Can you work these out from the model? Positions are in its coordinate system, mm. Coordinates: 2 decimals unless noted, no trailing zeros. Loops run counter-clockwise (first coordinate to the right, second up) from the corner with the lowest first, then second, coordinate; pieces in that order, holes last.
```python
from build123d import *

# Parameters (mm, degrees)
F0_R     = 35
F0_R_2   = 3.771368
F1_DEPTH = 35
F2_DEPTH = 25


with BuildPart() as f1:
    # F0 (on Top) → F1 (new body)
    with BuildSketch(Plane.XY):
        Circle(F0_R)
        with Locations((-0.389893, -27.902429)):
            Circle(F0_R_2, mode=Mode.SUBTRACT)
        with Locations((-16.670046, -22.486003)):
            Circle(F0_R_2, mode=Mode.SUBTRACT)
        with Locations((-26.65727, -8.534788)):
            Circle(F0_R_2, mode=Mode.SUBTRACT)
        with Locations((15.964723, -22.715176)):
            Circle(F0_R_2, mode=Mode.SUBTRACT)
        with Locations((26.146894, -8.905599)):
            Circle(F0_R_2, mode=Mode.SUBTRACT)
        with Locations((-26.536787, 8.622325)):
            Circle(F0_R_2, mode=Mode.SUBTRACT)
        with Locations((-16.354616, 22.431902)):
            Circle(F0_R_2, mode=Mode.SUBTRACT)
        with Locations((26.267377, 8.251514)):
            Circle(F0_R_2, mode=Mode.SUBTRACT)
        with Locations((16.280153, 22.202729)):
            Circle(F0_R_2, mode=Mode.SUBTRACT)
        with Locations((0, 27.619155)):
            Circle(F0_R_2, mode=Mode.SUBTRACT)
    extrude(amount=F1_DEPTH)

    # F0 (on Top) → F2 (join)
    with BuildSketch(Plane.XY):
        Circle(F0_R)
        with Locations((-0.389893, -27.902429)):
            Circle(F0_R_2, mode=Mode.SUBTRACT)
        with Locations((-16.670046, -22.486003)):
            Circle(F0_R_2, mode=Mode.SUBTRACT)
        with Locations((-26.65727, -8.534788)):
            Circle(F0_R_2, mode=Mode.SUBTRACT)
        with Locations((15.964723, -22.715176)):
            Circle(F0_R_2, mode=Mode.SUBTRACT)
        with Locations((26.146894, -8.905599)):
            Circle(F0_R_2, mode=Mode.SUBTRACT)
        with Locations((-26.536787, 8.622325)):
            Circle(F0_R_2, mode=Mode.SUBTRACT)
        with Locations((-16.354616, 22.431902)):
            Circle(F0_R_2, mode=Mode.SUBTRACT)
        with Locations((26.267377, 8.251514)):
            Circle(F0_R_2, mode=Mode.SUBTRACT)
        with Locations((16.280153, 22.202729)):
            Circle(F0_R_2, mode=Mode.SUBTRACT)
        with Locations((0, 27.619155)):
            Circle(F0_R_2, mode=Mode.SUBTRACT)
    extrude(amount=F2_DEPTH)


solid = f1.part
```
(1) I'm going to push flat-ended pins straight in: pin 1 (4 mm diameter, centred on y = -3, z = 6.5, fed in from +X); pin 2 (1.5 mm diameter, centred on x = -2.5, z = 30, fed in from +Y); pin 3 (5 mm diameter, centred on x = 2.5, z = 14, fed in from -Y). Where does each tip first touch, or does it pass through?
Check values:
pin 1: stops at x = 34.99
pin 2: stops at y = 34.96
pin 3: stops at y = -35
(2) I want a section at A-A on x = -14.5. Write out the boundary of the cut face in (y, z), then the cut area to 3 significant figures.
Check values:
outline: (-31.86, 0) - (-25.57, 0) - (-25.57, 35) - (-31.86, 35) - close; (-19.4, 0) - (19.15, 0) - (19.15, 35) - (-19.4, 35) - close; (25.72, 0) - (31.86, 0) - (31.86, 35) - (25.72, 35) - close
area: 1,780 mm2
(3) If I drill on probe 1 along Y at (x, z) = (0, 21); probe 2 along X at (y, z) = (11.5, 3); probe 3 along Y at (x, z) = (-16, 13), over which ranges is the centre line in solid material (lowest first)?
Check values:
probe 1: y = -35 to -31.65, -24.15 to 23.85, 31.39 to 35
probe 2: x = -33.06 to -28.97, -24.1 to 24.35, 28.18 to 33.06
probe 3: y = -31.13 to -26.2, -18.77 to 18.68, 26.19 to 31.13
(4) I want a section at C-C on x = 0. Write out the boundary of the cut face in (y, z).
Check values:
outline: (-35, 0) - (-31.65, 0) - (-31.65, 35) - (-35, 35) - close; (-24.15, 0) - (23.85, 0) - (23.85, 35) - (-24.15, 35) - close; (31.39, 0) - (35, 0) - (35, 35) - (31.39, 35) - close
(5) I want a section at B-B on z = 7.5. State how many separate pieces and enclosed holes the cut face has, then the cut area to 3 significant figures.
Check values:
separate pieces: 1
enclosed holes: 10
area: 3,400 mm2
(6) I want a section at D-D on y = -16. Write out the boundary of the cut face in (x, z).
Check values:
outline: (-31.13, 0) - (31.13, 0) - (31.13, 35) - (-31.13, 35) - close
(7) If we mould it in two halves opening along X, with no side actions, what happens to faces 1 (the cylindrical face through (19.45, -24.16, 17.26)), 2 (the cylindrical face through (-28, -21, 17)), 3 (the flat face through (0, 0, 35))? For each: released by +X, released by -X, zero draft, split by the parting line, or undercut.
Check values:
face 1: undercut
face 2: split by the parting line
face 3: zero draft
